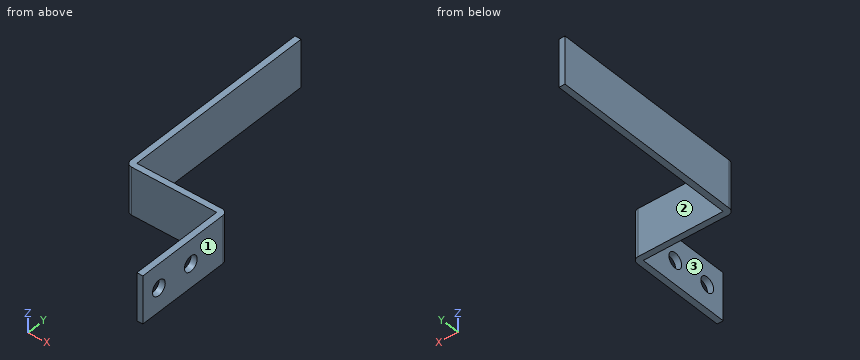
```python
from build123d import *

# Parameters (mm, degrees)
EXTRUDE_1_DEPTH          = 25
CUT_EXTRUDE_5_DEPTH      = 167.018071306
CUT_EXTRUDE_5_DEPTH_BACK = 167.018071306
SKETCH_7_R               = 4


with BuildPart() as part:
    # ｽｹｯﾁ1 → ﾎﾞｽ - 押し出し1 (new body)
    with BuildSketch(Plane.XY):
        with BuildLine():
            Line((0, 156), (0, 53.2))
            ThreePointArc((0, 53.2), (0.9372583, 50.9372583), (3.2, 50))
            Line((3.2, 50), (47.8, 50))
            Line((47.8, 50), (47.8, 0))
            Line((47.8, 0), (51, 0))
            Line((51, 0), (51, 50))
            ThreePointArc((51, 50), (50.0627417, 52.2627417), (47.8, 53.2))
            Line((47.8, 53.2), (3.2, 53.2))
            Line((3.2, 53.2), (3.2, 156))
            Line((3.2, 156), (0, 156))
        make_face()
    extrude(amount=EXTRUDE_1_DEPTH)

    # ｽｹｯﾁ7 → ｶｯﾄ - 押し出し5 (cut, two sides: drawn at the far end of the back side and taken through both)
    with BuildSketch(Plane(origin=(0, 0, 0), x_dir=(0, 0, -1), z_dir=(1, 0, 0)).offset(-CUT_EXTRUDE_5_DEPTH_BACK)):
        with Locations((-12.5, 10)):
            Circle(SKETCH_7_R)
        with Locations((-12.5, 30)):
            Circle(SKETCH_7_R)
    extrude(amount=CUT_EXTRUDE_5_DEPTH + CUT_EXTRUDE_5_DEPTH_BACK, mode=Mode.SUBTRACT)


solid = part.part
```
The listing builds one solid part. Answer for the finished solid, in the listing's coordinates (mm). Face numbers are marked on the shaded views. A direction names the side the tool comes from. Round coordinates to 2 decimals unless told otherwise and drop trailing zeros. Loops run counter-clockwise (first coordinate to the right, second up) from the corner with the lowest first, then second, coordinate; pieces in that order, holes last.
1) A cutting plane is placed at A-A on z = 12.5. Determine the outline of the cut face in (x, y).
Outcome:
outline: (0, 53.2) arc R3.2 ccw to (3.2, 50) - (47.8, 50) - (47.8, 34) - (51, 34) - (51, 50) arc R3.2 ccw to (47.8, 53.2) - (3.2, 53.2) - (3.2, 156) - (0, 156) - close; (47.8, 0) - (51, 0) - (51, 6) - (47.8, 6) - close; (47.8, 14) - (51, 14) - (51, 26) - (47.8, 26) - close
2) Consider line 1 (Y direction, x = 49.7, z = 12.5); line 2 (Z direction, x = 48.85, y = 30); line 3 (Y direction, x = 49.9, z = 12.5). Determine where each line is inside the solid, lowest interval first.
Outcome:
line 1: y = 0 to 6, 14 to 26, 34 to 52.57
line 2: z = 0 to 8.5, 16.5 to 25
line 3: y = 0 to 6, 14 to 26, 34 to 52.41
3) Given P1, Ø5, axis at x = 14.5, z = 13, coming from the +Y side; P2, Ø1.5, axis at y = 54.5, z = 5, coming from the +X side; P3, Ø9, axis at y = 30, z = 12.5, coming from the -X side, each flat-ended and moving along its own axis, determine where each tip first touches the part or whether it passes through.
Outcome:
P1: stops at y = 53.2
P2: stops at x = 3.2
P3: stops at x = 47.8
4) A cutting plane is placed at B-B on y = 10. Determine the outline of the cut face in (x, z), plus the area to 3 significant figures.
Outcome:
outline: (47.8, 0) - (51, 0) - (51, 8.5) - (47.8, 8.5) - close; (47.8, 16.5) - (51, 16.5) - (51, 25) - (47.8, 25) - close
area: 54.4 mm2
5) A cutting plane is placed at C-C on z = 5.75. Determine the outline of the cut face in (x, y), plus the area to 3 significant figures.
Outcome:
outline: (0, 53.2) arc R3.2 ccw to (3.2, 50) - (47.8, 50) - (47.8, 0) - (51, 0) - (51, 50) arc R3.2 ccw to (47.8, 53.2) - (3.2, 53.2) - (3.2, 156) - (0, 156) - close
area: 648 mm2
6) For the marked faces 1, 2 and 3, determine the directions among +Z, -Z, +X, -X, +Y, -Y from which every point of the face is accessible in a straight line to the end or side of a thin tool.
Outcome:
face 1: +Z, -Z, +X, +Y, -Y
face 2: +Z, -Z, +X, +Y
face 3: +Z, -Z, -X, -Y
7) A cutting plane is placed at D-D on x = 11. Determine the outline of the cut face in (y, z), plus the area to 3 significant figures.
Outcome:
outline: (50, 0) - (53.2, 0) - (53.2, 25) - (50, 25) - close
area: 80.0 mm2
